```python
from build123d import *

# Parameters (mm, degrees)
F1_DEPTH = 63.5
F2_DEPTH = 25.4
F3_DEPTH = 7.9375
F0_W     = 25.4
F0_H     = 19.05
F4_DEPTH = 63.5
F6_R     = 6.35


with BuildPart() as f1:
    # F0 (on Front) → F1 (new body, symmetric)
    with BuildSketch(Plane.XZ):
        Polygon((-41.275, 9.525), (-41.275, -9.525), (41.275, -9.525), (41.275, 9.525), (22.225, 9.525), align=None)
    extrude(amount=F1_DEPTH, both=True)

    # F0 (on Front) → F2 (join, symmetric)
    with BuildSketch(Plane.XZ):
        with BuildLine():
            Line((22.225, 9.525), (41.275, 9.525))
            Line((41.275, 9.525), (41.275, 27.0002))
            ThreePointArc((41.275, 27.0002), (45.9246798487, 38.2255201513), (57.15, 42.8752))
            Line((57.15, 42.8752), (60.325, 42.8752))
            Line((60.325, 42.8752), (60.325, 61.9252))
            Line((60.325, 61.9252), (57.15, 61.9252))
            ThreePointArc((57.15, 61.9252), (32.4542956671, 51.6959043329), (22.225, 27.0002))
            Line((22.225, 27.0002), (22.225, 9.525))
        make_face()
    extrude(amount=F2_DEPTH, both=True)

    # F0 (on Front) → F3 (join, symmetric)
    with BuildSketch(Plane.XZ):
        with BuildLine():
            add(Edge.make_bspline(
                [(-41.275, 9.525), (-23.7557739019, 48.5848635435), (20.1313588768, 70.8134099841), (57.15, 61.9252)],
                knots=[0, 0, 0, 0, 111.5045361635, 111.5045361635, 111.5045361635, 111.5045361635], degree=3))
            Line((-41.275, 9.525), (22.225, 9.525))
            Line((22.225, 9.525), (22.225, 27.0002))
            ThreePointArc((22.225, 27.0002), (32.4542956671, 51.6959043329), (57.15, 61.9252))
        make_face()
    extrude(amount=F3_DEPTH, both=True)

    # F0 (on Front) → F4 (join, symmetric)
    with BuildSketch(Plane.XZ):
        with Locations((73.025, 52.4002)):
            Rectangle(F0_W, F0_H)
    extrude(amount=F4_DEPTH, both=True)

    # F0 (on Front) → F5 (revolve)
    with BuildSketch(Plane.XZ):
        Polygon((85.725, 66.675), (85.725, 61.9252), (85.725, 42.8752), (85.725, 38.1), (111.125, 38.1), (111.125, 66.675), align=None)
    revolve(axis=Axis((85.725, 0, 52.3875), (0, 0, 1)))

    # F6
    f6_edges = [f1.edges().sort_by_distance(p)[0] for p in [
        (-41.275, -63.5, 0),
        (41.275, -63.5, 0),
        (41.275, 63.5, 0),
        (-41.275, 63.5, 0),
    ]]
    fillet(f6_edges, radius=F6_R)


solid = f1.part
```
Verification items for the finished model (mm, model axes). A direction names the side the tool comes from. Round coordinates to 2 decimals unless told otherwise and drop trailing zeros. Order: outer loops, then holes, each group sorted by start corner. A loop starts at its lowest first (then second) coordinate and runs counter-clockwise, first axis right, second up. Notation, with made-up numbers: (81.5, 77.25) -> (138.5, 77.25) arc R12 ccw to (138.5, 100.25) -> close; hole circle Ø9 at (23, 35). An arc over 180 degrees is marked (long way). Put each result on its own line as item: value. Start each with the question number.
(1) Depth check by flat-ended pin: pin 1 Ø9.5 at (y, z) = (49, 47.5) entering from -X (3 decimals); pin 2 Ø21 at (y, z) = (46.5, 48) entering from +X (3 decimals); pin 3 Ø15 at (x, y) = (91.5, 10) entering from -Z. Enter the tip coordinate at first touch or a pass-through.
(2) Section check A-A (y = -39.5). Enter the section's corners in (x, z) (3 decimals), then the cut area to 3 significant figures.
(3) Material ranges on line 1 along X through (y, z) = (57.5, -0.5); line 2 along Y through (x, z) = (-11, 23); line 3 along Y through (x, z) = (49, 44.5), recorded low to high.
(4) Section check B-B (z = -1). Enter the section's corners in (x, y) (3 decimals).
(5) Section check C-C (y = 21.5). Enter the section's corners in (x, z) (3 decimals).
(6) Tool access check on faces 1 (the face through (60.325, 44, 52)), 2 (the face through (60.325, -45, 52)), 3 (the face through (-2, -7.938, 34)), 4 (the face through (86, 0, 38.1)), 5 (the face through (-2, 7.938, 34)). Record the directions out of +Z, -Z, +X, -X, +Y, -Y that give a thin tool (end or side, any length) a straight path to the whole face; none if there is none.
Completed:
1. pin 1: stops at x = 60.325
1. pin 2: stops at x = 85.725
1. pin 3: stops at z = 38.1
2. outline: (-41.275, -9.525) -> (41.275, -9.525) -> (41.275, 9.525) -> (-41.275, 9.525) -> close; (60.325, 42.875) -> (85.725, 42.875) -> (85.725, 61.925) -> (60.325, 61.925) -> close
2. area: 2,060 mm2
3. line 1: x = -41.27 to 41.27
3. line 2: y = -7.94 to 7.94
3. line 3: y = -25.4 to 25.4
4. outline: (-41.275, -57.15) arc R6.35 ccw to (-34.925, -63.5) -> (34.925, -63.5) arc R6.35 ccw to (41.275, -57.15) -> (41.275, 57.15) arc R6.35 ccw to (34.925, 63.5) -> (-34.925, 63.5) arc R6.35 ccw to (-41.275, 57.15) -> close
5. outline: (-41.275, -9.525) -> (41.275, -9.525) -> (41.275, 27) arc R15.875 cw to (57.15, 42.875) -> (72.201, 42.875) -> (72.201, 38.1) -> (99.249, 38.1) -> (99.249, 66.675) -> (72.201, 66.675) -> (72.201, 61.925) -> (57.15, 61.925) arc R34.925 ccw to (22.225, 27) -> (22.225, 9.525) -> (-41.275, 9.525) -> close
6. face 1: +Z, -Z, -X, +Y
6. face 2: +Z, -Z, -X, -Y
6. face 3: +Z, -X, -Y
6. face 4: -Z, +X, +Y, -Y
6. face 5: +Z, -X, +Y
